```python
from build123d import *

# Parameters (mm, degrees)
SKETCH1_R               = 15.875
SKETCH1_R_2             = 13.462
BOSS_EXTRUDE1_DEPTH     = 30
CUT_EXTRUDE1_DEPTH      = 30
CUT_EXTRUDE1_DEPTH_BACK = 30
SKETCH2_R               = 2.25


with BuildPart() as part:
    # Sketch1 → Boss-Extrude1 (new body)
    with BuildSketch(Plane(origin=(0, 0, 0), x_dir=(1, 0, 0), z_dir=(0, 1, 0))):
        with Locations(Location((0, 0, 0), (0, 0, 270))):
            Circle(SKETCH1_R)
        with Locations(Location((0, 0, 0), (0, 0, 270))):
            Circle(SKETCH1_R_2, mode=Mode.SUBTRACT)
    extrude(amount=-BOSS_EXTRUDE1_DEPTH)

    # Sketch2 → Cut-Extrude1 (cut, two sides: drawn at the far end of the back side and taken through both)
    with BuildSketch(Plane.XY.offset(-CUT_EXTRUDE1_DEPTH_BACK)):
        with Locations(Location((0, -25, 0), (0, 0, 180))):
            Circle(SKETCH2_R)
        with Locations(Location((0, -10, 0), (0, 0, 180))):
            Circle(SKETCH2_R)
    extrude(amount=CUT_EXTRUDE1_DEPTH + CUT_EXTRUDE1_DEPTH_BACK, mode=Mode.SUBTRACT)


solid = part.part
```
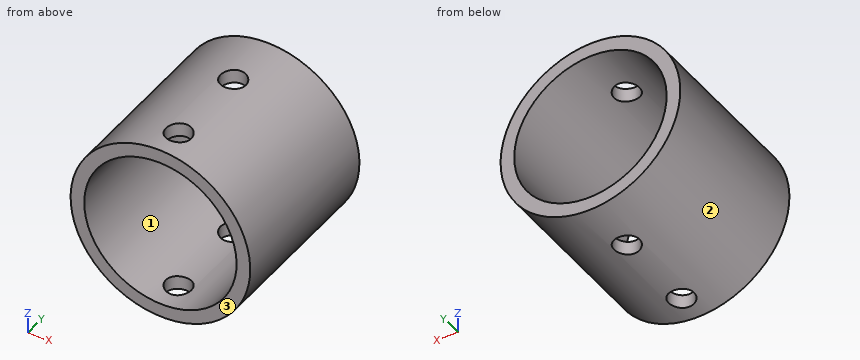
Part model, mm, in its own coordinate system. Face numbers are marked on the shaded views. Round coordinates to 2 decimals unless told otherwise and drop trailing zeros. Loops run counter-clockwise (first coordinate to the right, second up) from the corner with the lowest first, then second, coordinate; pieces in that order, holes last.
1. Slice it at D-D (y = -18). Give the cut face in (x, z) (3 decimals).
Solutions:
outline: circle Ø31.75 at (0, 0); hole circle Ø26.924 at (0, 0)
2. Slice it at C-C (x = 10). Give the cut face in (y, z).
Solutions:
outline: (-30, -12.33) - (0, -12.33) - (0, -9.01) - (-30, -9.01) - close; (-30, 9.01) - (0, 9.01) - (0, 12.33) - (-30, 12.33) - close
3. Slice it at A-A (z = 0). Give the cut face in (x, y) (3 decimals).
Solutions:
outline: (-15.875, -30) - (-13.462, -30) - (-13.462, 0) - (-15.875, 0) - close; (13.462, -30) - (15.875, -30) - (15.875, 0) - (13.462, 0) - close
4. Two-plate mould, pull along Z, no slides. Class the marked faces 1, 2 and 3: pulls with the +Z half, pulls with the -Z half, needs draft (parallel to the pull), parting line crosses it, or undercut.
Solutions:
face 1: undercut
face 2: parting line crosses it
face 3: needs draft
5. Flat gauge pins, fed straight in: pin 1 (3 mm diameter, centred on y = -20, z = -10.5, fed in from -X); pin 2 (4 mm diameter, centred on x = 0, y = -25, fed in from +Z); pin 3 (4 mm diameter, centred on x = 8, y = -12.5, fed in from -Z); pin 4 (12 mm diameter, centred on x = -9, y = -20, fed in from -Z). Where does each tip first touch, or does it go through?
Solutions:
pin 1: stops at x = -13.08
pin 2: passes through
pin 3: stops at z = -14.7
pin 4: stops at z = -15.59
6. Slice it at B-B (x = 0). Give the cut face in (y, z) (3 decimals), and give its area (3 significant figures).
Solutions:
outline: (-30, -15.875) - (-27.25, -15.875) - (-27.25, -13.462) - (-30, -13.462) - close; (-30, 13.462) - (-27.25, 13.462) - (-27.25, 15.875) - (-30, 15.875) - close; (-22.75, -15.875) - (-12.25, -15.875) - (-12.25, -13.462) - (-22.75, -13.462) - close; (-22.75, 13.462) - (-12.25, 13.462) - (-12.25, 15.875) - (-22.75, 15.875) - close; (-7.75, -15.875) - (0, -15.875) - (0, -13.462) - (-7.75, -13.462) - close; (-7.75, 13.462) - (0, 13.462) - (0, 15.875) - (-7.75, 15.875) - close
area: 101 mm2
7. Drill centre lines: line 1 along Y through (x, z) = (0, 14.1); line 2 along Z through (x, y) = (0, -16) (3 decimals). Where is each one in solid material? Low to high.
Solutions:
line 1: y = -30 to -27.25, -22.75 to -12.25, -7.75 to 0
line 2: z = -15.875 to -13.462, 13.462 to 15.875
